```python
from build123d import *

# Parameters (mm, degrees)
SKETCH1_W                      = 204.24
SKETCH1_H                      = 47.5
BOSS_EXTRUDE1_DEPTH            = 2.25
F_8_CLEARANCE_HOLE1_D          = 4.4958
FILLET1_R                      = 2
F_3_CLEARANCE_HOLE1_D          = 2.794
F_2_0_221_DIAMETER_HOLE1_D     = 2.50000008
F_2_0_221_DIAMETER_HOLE1_DEPTH = 20
F_2_0_221_DIAMETER_HOLE1_TIP   = 0.751075798


with BuildPart() as part:
    # Sketch1 → Boss-Extrude1 (new, symmetric)
    with BuildSketch(Plane.XY):
        Rectangle(SKETCH1_W, SKETCH1_H)
    extrude(amount=BOSS_EXTRUDE1_DEPTH, both=True)

    # #8 Clearance Hole1 (through all)
    with Locations(Plane.XY.offset(2.25)):
        with Locations((-82.12, 0)):
            Hole(F_8_CLEARANCE_HOLE1_D / 2)

    # Fillet1
    fillet1_edges = [part.edges().sort_by_distance(p)[0] for p in [
        (-102.12, 23.75, 0),
        (102.12, 23.75, 0),
        (102.12, -23.75, 0),
        (-102.12, -23.75, 0),
    ]]
    fillet(fillet1_edges, radius=FILLET1_R)

    # #3 Clearance Hole1 (through all)
    with Locations(Plane.XY.offset(2.25)):
        with Locations((-92.82, 10), (-92.82, -10)):
            Hole(F_3_CLEARANCE_HOLE1_D / 2)

    # #2 (0.221) Diameter Hole1
    with Locations(Plane(origin=(0, 0, -2.25), x_dir=(-1, 0, 0), z_dir=(0, 0, -1))):
        with Locations((-96.666875, 7.9375), (-96.666875, -7.9375)):
            Hole(F_2_0_221_DIAMETER_HOLE1_D / 2, depth=F_2_0_221_DIAMETER_HOLE1_DEPTH)
            with Locations((0, 0, -(F_2_0_221_DIAMETER_HOLE1_DEPTH + F_2_0_221_DIAMETER_HOLE1_TIP / 2))):  # 118° drill point
                Cone(0, F_2_0_221_DIAMETER_HOLE1_D / 2, F_2_0_221_DIAMETER_HOLE1_TIP, mode=Mode.SUBTRACT)


solid = part.part
```
Build history of the part. All positions in model axes, mm. Round coordinates to 2 decimals unless told otherwise and drop trailing zeros. Write each loop counter-clockwise with the first axis right and the second up, starting at its lowest first coordinate (ties: lowest second). Pieces come first, ordered by that corner, then holes.
1) Mould opens along Y. For faces 1 (the flat face through (-1, 23.75, 0)), 2 (the flat face through (-1, -23.75, 0)), 3 (the cylindrical face through (-84.264, 0.675, -0.031)) say: +Y half, -Y half, draft (parallel to the pull), parting line (faces both ways), or undercut.
2) Band-saw the part on B-B, the plane x = -82.12. List the corners of the cut face in (y, z), and give its area (3 significant figures).
3) Pin check, flat tip, straight feed: pin 1 (2 mm diameter, centred on x = -92.82, y = 10, fed in from +Z). Stop position of the tip, or through.
4) Drill centre lines: probe 1 along Y at (x, z) = (-92.82, 0.3); probe 2 along X at (y, z) = (9, -1.6); probe 3 along X at (y, z) = (7.5, -0.15). Where is each one in solid material? Low to high.
5) Band-saw the part on A-A, the plane y = 0. List the corners of the cut face in (x, z).
Ans:
1. face 1: +Y half
1. face 2: -Y half
1. face 3: undercut
2. outline: (-23.75, -2.25) - (-2.25, -2.25) - (-2.25, 2.25) - (-23.75, 2.25) - close; (2.25, -2.25) - (23.75, -2.25) - (23.75, 2.25) - (2.25, 2.25) - close
2. area: 194 mm2
3. pin 1: passes through
4. probe 1: y = -23.75 to -11.4, -8.6 to 8.6, 11.4 to 23.75
4. probe 2: x = -102.12 to -93.8, -91.84 to 96.01, 97.33 to 102.12
4. probe 3: x = -102.12 to 95.5, 97.84 to 102.12
5. outline: (-102.12, -2.25) - (-84.37, -2.25) - (-84.37, 2.25) - (-102.12, 2.25) - close; (-79.87, -2.25) - (102.12, -2.25) - (102.12, 2.25) - (-79.87, 2.25) - close
